For this review, take the finished solid that the model builds, in its own axes (mm). A direction names the side the tool comes from. Coordinates: 2 decimals unless noted, no trailing zeros. Write each loop counter-clockwise with the first axis right and the second up, starting at its lowest first coordinate (ties: lowest second). Pieces come first, ordered by that corner, then holes.
1) We need section C-C on y = -33.5. Write out the cut boundary in (x, z).
2) Mouldability with a two-part tool opening along Y and no side actions: class faces 1 (the face through (46.2, 7.629, 9.7)), 2 (the face through (44, -3.237, 13)), 3 (the face through (50.7, 5.4, 11.48)) as pulls with the +Y half, pulls with the -Y half, needs draft (parallel to the pull), parting line crosses it, or undercut.
3) We need section B-B on x = 0. Write out the cut boundary in (y, z), then the cut area to 3 significant figures.
4) Insertion check: P1, Ø5, axis at x = 27, z = 10.5, coming from the +Y side; P2, Ø5.5, axis at x = 47.77, z = 12.7, coming from the -Y side; P3, Ø8, axis at x = -18.5, z = 12.5, coming from the -Y side; P4, Ø1.5, axis at x = 30.5, z = 21.5, coming from the -Y side. Each pin has a flat end and moves straight along its axis. Give the tip position at first contact, or say it passes through.
5) We need section A-A on z = 12.7. Write out the cut boundary in (x, y), then the cut area to 3 significant figures.
6) We need section D-D on z = 19.25. Write out the cut boundary in (x, y), then the cut area to 3 significant figures.
7) For faces 4 (the face through (44, 3.237, 13)), 5 (the face through (50.7, -5.46, 11.48)), 6 (the face through (46.1, -7.629, 9.7)), list the 3-axis set-ups (+Z, -Z, +X, -X, +Y, -Y) from which the entire face can be reached by the end or side of a thin tool; tool diameter is ignored.
8) To check wall thickness, follow line 1 along Y through (x, z) = (0, 8.25); line 2 along Y through (x, z) = (30, 16); line 3 along X through (y, z) = (24, 20). State the ranges of each line that lie inside material, in increasing order.
from build123d import *

# Parameters (mm, degrees)
F1_DEPTH = 25.4
F3_D     = 6.35
F4_R     = 1.839631


with BuildPart() as f1:
    # F0 (on Top) → F1 (new body)
    with BuildSketch(Plane.XY):
        with BuildLine():
            ThreePointArc((34.949522, 7.62886), (35.355888, 5.443324), (35.62572, 3.236768))
            Line((35.62572, 3.236768), (41.997912, 3.236768))
            ThreePointArc((41.997912, 3.236768), (41.769655, 5.440338), (41.425859, 7.62886))
            Line((41.425859, 7.62886), (34.949522, 7.62886))
        make_face()
        with BuildLine():
            ThreePointArc((34.949522, -7.62886), (-35.772456, 0), (34.949522, 7.62886))
            Line((34.949522, 7.62886), (41.425859, 7.62886))
            ThreePointArc((41.425859, 7.62886), (-42.122456, 0), (41.425859, -7.62886))
            Line((41.425859, -7.62886), (34.949522, -7.62886))
        make_face()
        with BuildLine():
            ThreePointArc((41.425859, 7.62886), (41.769655, 5.440338), (41.997912, 3.236768))
            Line((41.997912, 3.236768), (53.603914, 3.236768))
            Line((53.603914, 3.236768), (53.603914, 7.62886))
            Line((53.603914, 7.62886), (41.425859, 7.62886))
        make_face()
        with BuildLine():
            ThreePointArc((35.62572, -3.236768), (35.355888, -5.443324), (34.949522, -7.62886))
            Line((34.949522, -7.62886), (41.425859, -7.62886))
            ThreePointArc((41.425859, -7.62886), (41.769655, -5.440338), (41.997912, -3.236768))
            Line((41.997912, -3.236768), (35.62572, -3.236768))
        make_face()
        with BuildLine():
            ThreePointArc((41.997912, -3.236768), (41.769655, -5.440338), (41.425859, -7.62886))
            Line((41.425859, -7.62886), (53.603914, -7.62886))
            Line((53.603914, -7.62886), (53.603914, -3.236768))
            Line((53.603914, -3.236768), (41.997912, -3.236768))
        make_face()
    extrude(amount=F1_DEPTH)

    # F3 (through all)
    with Locations(Plane(origin=(0, 7.62886, 0), x_dir=(-1, 0, 0), z_dir=(0, 1, 0))):
        with Locations((-47.770534, 12.7)):
            Hole(F3_D / 2)

    # F4
    f4_edges = [f1.edges().sort_by_distance(p)[0] for p in [
        (53.603914, 3.236768, 12.7),
        (53.603914, -3.236768, 12.7),
    ]]
    fillet(f4_edges, radius=F4_R)


solid = f1.part
Result:
1. outline: (-25.54, 0) - (-12.55, 0) - (-12.55, 25.4) - (-25.54, 25.4) - close; (12.55, 0) - (25.54, 0) - (25.54, 25.4) - (12.55, 25.4) - close
2. face 1: pulls with the +Y half
2. face 2: undercut
2. face 3: needs draft
3. outline: (-42.12, 0) - (-35.77, 0) - (-35.77, 25.4) - (-42.12, 25.4) - close; (35.77, 0) - (42.12, 0) - (42.12, 25.4) - (35.77, 25.4) - close
3. area: 323 mm2
4. P1: stops at y = 34.26
4. P2: passes through
4. P3: stops at y = -39.55
4. P4: stops at y = -29.82
5. outline: (34.95, -7.63) arc R35.77 cw (long way) to (34.95, 7.63) arc R35.77 cw to (35.63, 3.24) - (44.6, 3.24) - (44.6, 7.63) - (41.43, 7.63) arc R42.12 ccw (long way) to (41.43, -7.63) - (44.6, -7.63) - (44.6, -3.24) - (35.63, -3.24) arc R35.77 cw to start; (50.95, -7.63) - (53.6, -7.63) - (53.6, -5.08) arc R1.84 ccw to (51.76, -3.24) - (50.95, -3.24) - close; (50.95, 3.24) - (51.76, 3.24) arc R1.84 ccw to (53.6, 5.08) - (53.6, 7.63) - (50.95, 7.63) - close
5. area: 1,560 mm2
6. outline: (34.95, -7.63) arc R35.77 cw (long way) to (34.95, 7.63) arc R35.77 cw to (35.63, 3.24) - (51.76, 3.24) arc R1.84 ccw to (53.6, 5.08) - (53.6, 7.63) - (41.43, 7.63) arc R42.12 ccw (long way) to (41.43, -7.63) - (53.6, -7.63) - (53.6, -5.08) arc R1.84 ccw to (51.76, -3.24) - (35.63, -3.24) arc R35.77 cw to start
6. area: 1,620 mm2
7. face 4: +Z, -Z, +X
7. face 5: +Y, -Y
7. face 6: +Z, -Z, +X, -Y
8. line 1: y = -42.12 to -35.77, 35.77 to 42.12
8. line 2: y = -29.57 to -19.49, 19.49 to 29.57
8. line 3: x = -34.62 to -26.53, 26.53 to 34.62
